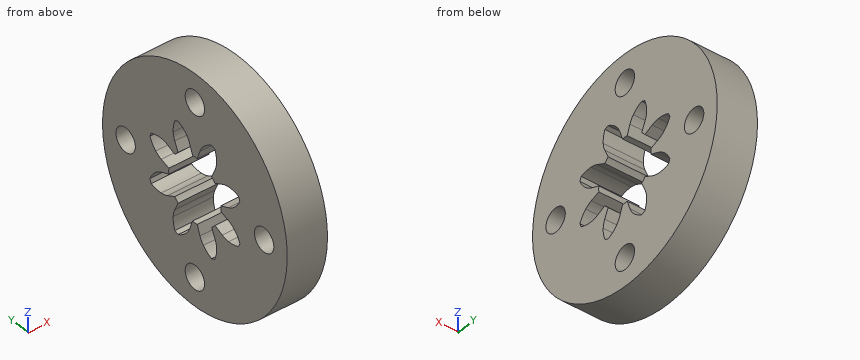
```python
from build123d import *

# Parameters (mm, degrees)
ESBO_O1_W             = 7.2
ESBO_O1_H             = 20
CORTE_EXTRUS_O2_DEPTH = 30.186298155
FURO_ROSCADO_DE_M51_D = 4.2


with BuildPart() as part:
    # Esboço1 → Revolução1 (revolve)
    with BuildSketch(Plane.XY, mode=Mode.PRIVATE) as revolu_o1_sk:
        with Locations((3.6, 10)):
            Rectangle(ESBO_O1_W, ESBO_O1_H)
    revolve(revolu_o1_sk.sketch.rotate(Axis((-35, 0, 0), (1, 0, 0)), 90), axis=Axis((-35, 0, 0), (1, 0, 0)))

    # Esboço3 → Corte-extrusão2 (cut, through all)
    with BuildSketch(Plane(origin=(7.2, 0, 0), x_dir=(0, 0, -1), z_dir=(1, 0, 0))):
        with BuildLine():
            Line((-0.506751832, 5.642289215), (-1.097919721, 7.266509641))
            ThreePointArc((-1.097919721, 7.266509641), (-1.406126414, 7.910707201), (-1.832951119, 8.483247621))
            ThreePointArc((-1.832951119, 8.483247621), (-2.661618953, 9.214061597), (-3.630088541, 9.745894376))
            ThreePointArc((-3.630088541, 9.745894376), (-3.979907697, 9.608347138), (-4.324527778, 9.458248225))
            ThreePointArc((-4.324527778, 9.458248225), (-4.633276627, 8.397374248), (-4.702469753, 7.294654085))
            ThreePointArc((-4.702469753, 7.294654085), (-4.599433183, 6.587996228), (-4.361851763, 5.914544723))
            Line((-4.361851763, 5.914544723), (-3.631373309, 4.348028622))
            ThreePointArc((-3.631373309, 4.348028622), (-4.005759915, 4.005759915), (-4.348028622, 3.631373309))
            Line((-4.348028622, 3.631373309), (-5.914544723, 4.361851763))
            ThreePointArc((-5.914544723, 4.361851763), (-6.587996228, 4.599433183), (-7.294654085, 4.702469753))
            ThreePointArc((-7.294654085, 4.702469753), (-8.397374248, 4.633276627), (-9.458248225, 4.324527778))
            ThreePointArc((-9.458248225, 4.324527778), (-9.608347138, 3.979907697), (-9.745894376, 3.630088541))
            ThreePointArc((-9.745894376, 3.630088541), (-9.214061597, 2.661618953), (-8.483247621, 1.832951119))
            ThreePointArc((-8.483247621, 1.832951119), (-7.910707201, 1.406126414), (-7.266509641, 1.097919721))
            Line((-7.266509641, 1.097919721), (-5.642289215, 0.506751832))
            ThreePointArc((-5.642289215, 0.506751832), (-5.665, 0), (-5.642289215, -0.506751832))
            Line((-5.642289215, -0.506751832), (-7.266509641, -1.097919721))
            ThreePointArc((-7.266509641, -1.097919721), (-7.910707201, -1.406126414), (-8.483247621, -1.832951119))
            ThreePointArc((-8.483247621, -1.832951119), (-9.214061597, -2.661618953), (-9.745894376, -3.630088541))
            ThreePointArc((-9.745894376, -3.630088541), (-9.608347138, -3.979907697), (-9.458248225, -4.324527778))
            ThreePointArc((-9.458248225, -4.324527778), (-8.397374248, -4.633276627), (-7.294654085, -4.702469753))
            ThreePointArc((-7.294654085, -4.702469753), (-6.587996228, -4.599433183), (-5.914544723, -4.361851763))
            Line((-5.914544723, -4.361851763), (-4.348028622, -3.631373309))
            ThreePointArc((-4.348028622, -3.631373309), (-4.005759915, -4.005759915), (-3.631373309, -4.348028622))
            Line((-3.631373309, -4.348028622), (-4.361851763, -5.914544723))
            ThreePointArc((-4.361851763, -5.914544723), (-4.599433183, -6.587996228), (-4.702469753, -7.294654085))
            ThreePointArc((-4.702469753, -7.294654085), (-4.633276627, -8.397374248), (-4.324527778, -9.458248225))
            ThreePointArc((-4.324527778, -9.458248225), (-3.979907697, -9.608347138), (-3.630088541, -9.745894376))
            ThreePointArc((-3.630088541, -9.745894376), (-2.661618953, -9.214061597), (-1.832951119, -8.483247621))
            ThreePointArc((-1.832951119, -8.483247621), (-1.406126414, -7.910707201), (-1.097919721, -7.266509641))
            Line((-1.097919721, -7.266509641), (-0.506751832, -5.642289215))
            ThreePointArc((-0.506751832, -5.642289215), (0, -5.665), (0.506751832, -5.642289215))
            Line((0.506751832, -5.642289215), (1.097919721, -7.266509641))
            ThreePointArc((1.097919721, -7.266509641), (1.406126414, -7.910707201), (1.832951119, -8.483247621))
            ThreePointArc((1.832951119, -8.483247621), (2.661618953, -9.214061597), (3.630088541, -9.745894376))
            ThreePointArc((3.630088541, -9.745894376), (3.979907697, -9.608347138), (4.324527778, -9.458248225))
            ThreePointArc((4.324527778, -9.458248225), (4.633276627, -8.397374248), (4.702469753, -7.294654085))
            ThreePointArc((4.702469753, -7.294654085), (4.599433183, -6.587996228), (4.361851763, -5.914544723))
            Line((4.361851763, -5.914544723), (3.631373309, -4.348028622))
            ThreePointArc((3.631373309, -4.348028622), (4.005759915, -4.005759915), (4.348028622, -3.631373309))
            Line((4.348028622, -3.631373309), (5.914544723, -4.361851763))
            ThreePointArc((5.914544723, -4.361851763), (6.587996228, -4.599433183), (7.294654085, -4.702469753))
            ThreePointArc((7.294654085, -4.702469753), (8.397374248, -4.633276627), (9.458248225, -4.324527778))
            ThreePointArc((9.458248225, -4.324527778), (9.608347138, -3.979907697), (9.745894376, -3.630088541))
            ThreePointArc((9.745894376, -3.630088541), (9.214061597, -2.661618953), (8.483247621, -1.832951119))
            ThreePointArc((8.483247621, -1.832951119), (7.910707201, -1.406126414), (7.266509641, -1.097919721))
            Line((7.266509641, -1.097919721), (5.642289215, -0.506751832))
            ThreePointArc((5.642289215, -0.506751832), (5.665, 0), (5.642289215, 0.506751832))
            Line((5.642289215, 0.506751832), (7.266509641, 1.097919721))
            ThreePointArc((7.266509641, 1.097919721), (7.910707201, 1.406126414), (8.483247621, 1.832951119))
            ThreePointArc((8.483247621, 1.832951119), (9.214061597, 2.661618953), (9.745894376, 3.630088541))
            ThreePointArc((9.745894376, 3.630088541), (9.608347138, 3.979907697), (9.458248225, 4.324527778))
            ThreePointArc((9.458248225, 4.324527778), (8.397374248, 4.633276627), (7.294654085, 4.702469753))
            ThreePointArc((7.294654085, 4.702469753), (6.587996228, 4.599433183), (5.914544723, 4.361851763))
            Line((5.914544723, 4.361851763), (4.348028622, 3.631373309))
            ThreePointArc((4.348028622, 3.631373309), (4.005759915, 4.005759915), (3.631373309, 4.348028622))
            Line((3.631373309, 4.348028622), (4.361851763, 5.914544723))
            ThreePointArc((4.361851763, 5.914544723), (4.599433183, 6.587996228), (4.702469753, 7.294654085))
            ThreePointArc((4.702469753, 7.294654085), (4.633276627, 8.397374248), (4.324527778, 9.458248225))
            ThreePointArc((4.324527778, 9.458248225), (3.979907697, 9.608347138), (3.630088541, 9.745894376))
            ThreePointArc((3.630088541, 9.745894376), (2.661618953, 9.214061597), (1.832951119, 8.483247621))
            ThreePointArc((1.832951119, 8.483247621), (1.406126414, 7.910707201), (1.097919721, 7.266509641))
            Line((1.097919721, 7.266509641), (0.506751832, 5.642289215))
            ThreePointArc((0.506751832, 5.642289215), (0, 5.665), (-0.506751832, 5.642289215))
        make_face()
    extrude(amount=-CORTE_EXTRUS_O2_DEPTH, mode=Mode.SUBTRACT)

    # Furo roscado de M51 (through all)
    with Locations(Plane(origin=(7.2, 0, 0), x_dir=(0, 0, -1), z_dir=(1, 0, 0))):
        with Locations((0, 15), (15, 0), (0, -15), (-15, 0)):
            Hole(FURO_ROSCADO_DE_M51_D / 2)


solid = part.part
```
Check sheet for the modelled part. Datum: model origin and axes. Units: mm. Round coordinates to 2 decimals unless told otherwise and drop trailing zeros. Order: outer loops, then holes, each group sorted by start corner. A loop starts at its lowest first (then second) coordinate and runs counter-clockwise, first axis right, second up.
1) Section check A-A (y = 0). Record the boundary of the cut face in (x, z) (3 decimals).
2) Section check D-D (x = 0.5). Give the number of separate pieces and of enclosed holes in the cut face, and give its area (3 significant figures).
3) Section check B-B (z = -15). Record the boundary of the cut face in (x, y).
4) Scan lines: line 1 (Z direction, x = 5, y = 6); line 2 (Z direction, x = 2.5, y = 7) (3 decimals); line 3 (Y direction, x = 6.25, z = 7.5). Record each from-to range of solid material in increasing order.
5) Go/stop test with flat-tipped pins: pin 1 Ø3 at (x, y) = (6.5, 9.5) entering from -Z; pin 2 Ø1 at (x, y) = (1, -10.5) entering from -Z; pin 3 Ø1 at (x, z) = (4.5, 11.5) entering from -Y; pin 4 Ø1.5 at (y, z) = (-13.5, -11.5) entering from -X. Record where each tip stops, or that it passes through.
Result:
1. outline: (0, -20) - (7.2, -20) - (7.2, -17.1) - (0, -17.1) - close; (0, -12.9) - (7.2, -12.9) - (7.2, -5.665) - (0, -5.665) - close; (0, 5.665) - (7.2, 5.665) - (7.2, 12.9) - (0, 12.9) - close; (0, 17.1) - (7.2, 17.1) - (7.2, 20) - (0, 20) - close
2. separate pieces: 1
2. enclosed holes: 5
2. area: 987 mm2
3. outline: (0, -13.23) - (7.2, -13.23) - (7.2, -2.1) - (0, -2.1) - close; (0, 2.1) - (7.2, 2.1) - (7.2, 13.23) - (0, 13.23) - close
4. line 1: z = -19.08 to -4.4, -0.64 to 0.64, 4.4 to 19.08
4. line 2: z = -18.735 to -4.677, -1.001 to 1.001, 4.677 to 18.735
4. line 3: y = -18.54 to -4.71, -1.19 to 1.19, 4.71 to 18.54
5. pin 1: stops at z = -18.33
5. pin 2: stops at z = -17.32
5. pin 3: stops at y = -16.7
5. pin 4: stops at x = 0
